Source: CAD feature listing. Evaluate the final solid. Frame: model axes, mm. Give positions to 0.01 mm unless a question says otherwise; leave off trailing zeros. Order: outer loops, then holes, each group sorted by start corner. A loop starts at its lowest first (then second) coordinate and runs counter-clockwise, first axis right, second up. Notation, with made-up numbers: M 67.25,35 L 88.25,35 A30 ccw 88.25,63 Z; hole C 73,-8 d10. An arc over 180 degrees is marked long. Answer in a Markdown table with one row per item. Add a question column.
(1) Section query C-C, the plane y = -3.5. Return loops of the section in (x, z).
(2) Pin query (flat end, axial travel): P1, Ø2, axis at x = 2, z = -7, coming from the -Y side; P2, Ø5, axis at y = 0, z = 15, coming from the -X side; P3, Ø1, axis at x = 1, z = 8, coming from the -Y side. Return the tip coordinate at first contact, or that it passes through.
(3) Section query A-A, the plane x = 3.6. Return loops of the section in (y, z), plus the area to 3 significant figures.
(4) Material intervals for line 1 along Z through (x, y) = (2.5, 1.75); line 2 along Z through (x, y) = (0.9, -3.75); line 3 along Y through (x, z) = (1.35, -3.5), sorted ascending.
(5) Section query D-D, the plane z = -33.5. Return loops of the section in (x, y).
(6) Mould query, pull axis Z, two halves, no side actions, for faces 1 (the face through (2.46, -1.73, -7.81)), 2 (the face through (2.46, -0.1, -49.55)), 3 (the face through (5, 0, -13)), 4 (the face through (2.46, -1.11, 16.01)). Classes: pulls with the +Z half, pulls with the -Z half, needs draft (parallel to the pull), parting line crosses it, or undercut.
(7) Section query B-B, the plane z = 15. Return loops of the section in (x, y), plus the area to 3 significant figures.
from build123d import *

# Parameters (mm, degrees)
F0_R     = 2.55
F0_R_2   = 8
F0_R_3   = 1.5
F1_DEPTH = 5


with BuildPart() as f1:
    # F0 (on Right) → F1 (new body)
    with BuildSketch(Plane.YZ):
        with BuildLine():
            Line((10.696365, 2.566667), (7.292976, 16.75))
            ThreePointArc((7.292976, 16.75), (0, 22.5), (-7.292976, 16.75))
            Line((-7.292976, 16.75), (-10.696365, 2.566667))
            ThreePointArc((-10.696365, 2.566667), (-10.986044, 0.553925), (-10.900287, -1.477746))
            Line((-10.900287, -1.477746), (-5, -45))
            ThreePointArc((-5, -45), (0, -49.55), (5, -45))
            Line((5, -45), (10.900287, -1.477746))
            ThreePointArc((10.900287, -1.477746), (10.986044, 0.553925), (10.696365, 2.566667))
        make_face()
        with Locations((0, -45)):
            Circle(F0_R, mode=Mode.SUBTRACT)
        Circle(F0_R_2, mode=Mode.SUBTRACT)
        with Locations((0, 15)):
            Circle(F0_R_3, mode=Mode.SUBTRACT)
    extrude(amount=F1_DEPTH)


solid = f1.part
Values follow:
| question | item | result |
|---|---|---|
| 1 | outline | M 0,-48.13 L 5,-48.13 L 5,-7.19 L 0,-7.19 Z; M 0,7.19 L 5,7.19 L 5,21.63 L 0,21.63 Z |
| 2 | P1 | stops at y = -10.29 |
| 2 | P2 | stops at x = 0 |
| 2 | P3 | stops at y = -9.51 |
| 3 | outline | M -10.9,-1.48 L -5,-45 A5.02 ccw 5,-45 L 10.9,-1.48 A11 ccw 10.7,2.57 L 7.29,16.75 A7.5 ccw -7.29,16.75 L -10.7,2.57 A11 ccw Z; hole C 0,0 d16; hole C 0,-45 d5.1; hole C 0,15 d3 |
| 3 | area | 904 mm² |
| 4 | line 1 | z = -49.24 to -46.85, -43.15 to -7.81, 7.81 to 22.29 |
| 4 | line 2 | z = -47.87 to -7.07, 7.07 to 21.5 |
| 4 | line 3 | y = -10.63 to -7.19, 7.19 to 10.63 |
| 5 | outline | M 0,-6.56 L 5,-6.56 L 5,6.56 L 0,6.56 Z |
| 6 | face 1 | undercut |
| 6 | face 2 | pulls with the -Z half |
| 6 | face 3 | needs draft |
| 6 | face 4 | undercut |
| 7 | outline | M 0,-7.71 L 5,-7.71 L 5,-1.5 L 0,-1.5 Z; M 0,1.5 L 5,1.5 L 5,7.71 L 0,7.71 Z |
| 7 | area | 62.1 mm² |
